```python
from build123d import *

# Parameters (mm, degrees)
F1_DEPTH = 25.4
F2_R     = 5.08
F3_R     = 5.08


with BuildPart() as f1:
    # F0 (on Top) → F1 (new body)
    with BuildSketch(Plane.XY):
        with BuildLine():
            ThreePointArc((-635, 117.375871), (-629.849929, -11.178382), (-635, -139.732635))
            Line((-635, -139.732635), (0, -139.732635))
            Line((0, -139.732635), (635, -139.732635))
            ThreePointArc((635, -139.732635), (629.849929, -11.178382), (635, 117.375871))
            Line((635, 117.375871), (0, 117.375871))
            Line((0, 117.375871), (-635, 117.375871))
        make_face()
        with BuildLine():
            ThreePointArc((-43.281963, 17.344755), (-46.751505, 47.124444), (-17.833089, 39.212882))
            Line((-17.833089, 39.212882), (-3.765872, 15.682267))
            ThreePointArc((-3.765872, 15.682267), (0.431929, 13.301076), (4.62973, 15.682267))
            Line((4.62973, 15.682267), (19.791877, 41.044401))
            ThreePointArc((19.791877, 41.044401), (46.275397, 47.39389), (48.414995, 20.24403))
            Line((48.414995, 20.24403), (17.154038, 2.016637))
            ThreePointArc((17.154038, 2.016637), (15.749838, -1.278464), (17.74202, -4.255153))
            Line((17.74202, -4.255153), (48.315184, -20.3542))
            ThreePointArc((48.315184, -20.3542), (49.888098, -48.459777), (21.858588, -45.862841))
            Line((21.858588, -45.862841), (6.283131, -19.133924))
            ThreePointArc((6.283131, -19.133924), (2.217899, -16.634052), (-1.847334, -19.133924))
            Line((-1.847334, -19.133924), (-13.774237, -42.722683))
            ThreePointArc((-13.774237, -42.722683), (-43.686922, -50.190632), (-42.133754, -19.398967))
            Line((-42.133754, -19.398967), (-15.645329, -4.420306))
            ThreePointArc((-15.645329, -4.420306), (-14.166998, -0.694867), (-15.645329, 3.030572))
            Line((-15.645329, 3.030572), (-43.281963, 17.344755))
        make_face(mode=Mode.SUBTRACT)
    extrude(amount=F1_DEPTH)

    # F2
    f2_edges = [f1.edges().sort_by_distance(p)[0] for p in [
        (-629.849929, -11.178382, 0),
    ]]
    fillet(f2_edges, radius=F2_R)

    # F3
    f3_edges = [f1.edges().sort_by_distance(p)[0] for p in [
        (629.849929, -11.178382, 0),
    ]]
    fillet(f3_edges, radius=F3_R)


solid = f1.part
```
Can you work these out from the model? Positions are in its coordinate system, mm. A direction names the side the tool comes from. Round coordinates to 2 decimals unless told otherwise and drop trailing zeros. Order: outer loops, then holes, each group sorted by start corner. A loop starts at its lowest first (then second) coordinate and runs counter-clockwise, first axis right, second up. Notation, with made-up numbers: (31.5, 88) -> (70.5, 88) arc R37 ccw to (70.5, 127) -> close; hole circle Ø7 at (18, 41.25). An arc over 180 degrees is marked (long way). Return JSON: item names as keys, results as strings. Group by question number.
1. If we section it at A-A, the plane z = 19: Write out the boundary of the cut face in (x, y) (1 decimal), then the cut area to 3 significant figures.
2. We'd pull the mould along X, two halves only. Please class faces 1 (the face through (-629.85, -9.38, 15.1)), 2 (the face through (-9, -38, 0)), 3 (the face through (50.206, -48.146, 12.522)): released by +X, released by -X, zero draft, split by the parting line, or undercut.
3. Which directions (+Z, -Z, +X, -X, +Y, -Y) give clear straight access to the entire face, cutting with the end or side of a thin tool? Please do faces 4 (the face through (-29.27, 10.087, 12.522)), 5 (the face through (629.85, -12.98, 15.1)).
4. I need wall thicknesses on line 1 (X direction, y = -26.5, z = 9.5); line 2 (X direction, y = 39, z = 13.25); line 3 (X direction, y = 1, z = 13). Which ranges of each line are inside material? Lowest first, please. Write a range as [from, to].
Output values:
{
 "1": {"outline": "(-635, -139.7) -> (635, -139.7) arc R1607 cw to (635, 117.4) -> (-635, 117.4) arc R1607 cw to start; hole (-43.3, 17.3) -> (-15.6, 3) arc R5.4 cw to (-15.6, -4.4) -> (-42.1, -19.4) arc R19.2 ccw (long way) to (-13.8, -42.7) -> (-1.8, -19.1) arc R4.6 cw to (6.3, -19.1) -> (21.9, -45.9) arc R18.6 ccw (long way) to (48.3, -20.4) -> (17.7, -4.3) arc R3.8 cw to (17.2, 2) -> (48.4, 20.2) arc R17.9 ccw (long way) to (19.8, 41) -> (4.6, 15.7) arc R4.9 cw to (-3.8, 15.7) -> (-17.8, 39.2) arc R18.1 ccw (long way) to start", "area": "318,000 mm²"},
 "2": {"face 1": "released by -X", "face 2": "zero draft", "face 3": "undercut"},
 "3": {"face 4": "+Z, -Z", "face 5": "+Z, -Z, +X"},
 "4": {"line 1": "[-629.92, -48.51], [-5.57, 10.58], [53.47, 629.92]", "line 2": "[-630.63, -52.16], [-17.71, 18.57], [52.59, 630.63]", "line 3": "[-629.9, -14.44], [16.26, 629.9]"}
}
